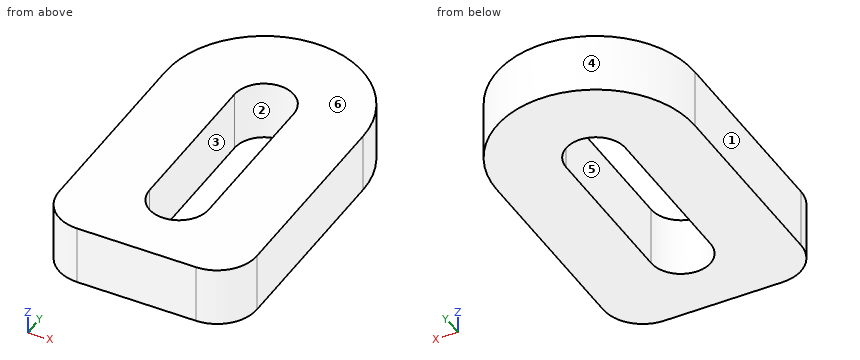
```python
from build123d import *

# Parameters (mm, degrees)
PAD_DEPTH = 3
FILLET_R  = 2


with BuildPart() as part:
    # Sketch → Pad (new body)
    with BuildSketch(Plane.XY):
        with BuildLine():
            ThreePointArc((5, 0), (0, 5), (-5, 0))
            Line((-5, 0), (-5, -12))
            Line((-5, -12), (5, -12))
            Line((5, -12), (5, 0))
        make_face()
        with BuildLine():
            ThreePointArc((1.5, 0), (0, 1.5), (-1.5, 0))
            Line((-1.5, 0), (-1.5, -8))
            ThreePointArc((-1.5, -8), (0, -9.5), (1.5, -8))
            Line((1.5, 0), (1.5, -8))
        make_face(mode=Mode.SUBTRACT)
    extrude(amount=PAD_DEPTH)

    # Fillet
    fillet_edges = [part.edges().sort_by_distance(p)[0] for p in [
        (-5, -12, 1.5),
        (5, -12, 1.5),
    ]]
    fillet(fillet_edges, radius=FILLET_R)


solid = part.part
```
The listing builds one solid part. Answer for the finished solid, in the listing's coordinates (mm). Face numbers are marked on the shaded views. A direction names the side the tool comes from. Round coordinates to 2 decimals unless told otherwise and drop trailing zeros. Loops run counter-clockwise (first coordinate to the right, second up) from the corner with the lowest first, then second, coordinate; pieces in that order, holes last. Notation, with made-up numbers: (-10, 53.25) - (18, 53.25) arc R15 ccw to (18, 66.25) - close; hole circle Ø8 at (59, 10.25). An arc over 180 degrees is marked (long way). Use one line per item in the form item = value. Start each with the question number.
1. The part is cut by section D-D on x = -3.5. Determine the outline of the cut face in (y, z).
2. The part is cut by section B-B on x = 0. Determine the outline of the cut face in (y, z).
3. Consider line 1 (X direction, y = -1.75, z = 2.4); line 2 (Y direction, x = 0, z = 2.8); line 3 (X direction, y = 1.25, z = 2.4). Determine where each line is inside the solid, lowest interval first. Write a range as [from, to].
4. A tool of negligible diameter and unlimited length cuts with its end or side. For the marked faces 5 and 6, from which of +Z, -Z, +X, -X, +Y, -Y can it reach the whole face along a straight path? Write none if from no direction.
5. For a pull along Y with two mould halves and no side action, classify the marked faces 1, 2, 3 and 4 as pulls with the +Y half, pulls with the -Y half, needs draft (parallel to the pull), parting line crosses it, or undercut.
6. The part is cut by section C-C on y = -2.5. Determine the outline of the cut face in (x, z), then the cut area to 3 significant figures.
7. The part is cut by section A-A on z = 1.9. Determine the outline of the cut face in (x, y).
Geometry check:
q1.outline = (-11.94, 0) - (3.57, 0) - (3.57, 3) - (-11.94, 3) - close
q2.outline = (-12, 0) - (-9.5, 0) - (-9.5, 3) - (-12, 3) - close; (1.5, 0) - (5, 0) - (5, 3) - (1.5, 3) - close
q3.line_1 = [-5, -1.5], [1.5, 5]
q3.line_2 = [-12, -9.5], [1.5, 5]
q3.line_3 = [-4.84, -0.83], [0.83, 4.84]
q4.face_5 = +Z, -Z
q4.face_6 = +Z, +X, -X, +Y, -Y
q5.face_1 = needs draft
q5.face_2 = undercut
q5.face_3 = undercut
q5.face_4 = pulls with the +Y half
q6.outline = (-5, 0) - (-1.5, 0) - (-1.5, 3) - (-5, 3) - close; (1.5, 0) - (5, 0) - (5, 3) - (1.5, 3) - close
q6.area = 21.0 mm^2
q7.outline = (-5, -10) arc R2 ccw to (-3, -12) - (3, -12) arc R2 ccw to (5, -10) - (5, 0) arc R5 ccw to (-5, 0) - close; hole (-1.5, -8) arc R1.5 ccw to (1.5, -8) - (1.5, 0) arc R1.5 ccw to (-1.5, 0) - close
